from build123d import *

# Parameters (mm, degrees)
SKETCH1_R           = 7.875
BOSS_EXTRUDE1_DEPTH = 20.68
SKETCH2_R           = 8.915
BOSS_EXTRUDE2_DEPTH = 2.03
SKETCH3_R           = 5.965
SKETCH3_R_2         = 5.215
CUT_EXTRUDE1_DEPTH  = 0.4
CHAMFER1_SIZE       = 1.2
CHAMFER1_SIZE2      = 2.6
SKETCH4_R           = 5.34
BOSS_EXTRUDE3_DEPTH = 8.7
SKETCH5_W           = 0.4
SKETCH5_H           = 1.86
BOSS_EXTRUDE4_DEPTH = 5.65
SKETCH6_R           = 0.5
CUT_EXTRUDE2_DEPTH  = 14.552865697
FILLET1_R           = 2


with BuildPart() as part:
    # Sketch1 → Boss-Extrude1 (new body)
    with BuildSketch(Plane(origin=(0, 0, 0), x_dir=(0, 0, -1), z_dir=(1, 0, 0))):
        Circle(SKETCH1_R)
    extrude(amount=BOSS_EXTRUDE1_DEPTH)

    # Sketch2 → Boss-Extrude2 (add)
    with BuildSketch(Plane(origin=(20.68, 0, 0), x_dir=(0, 0, -1), z_dir=(1, 0, 0))):
        Circle(SKETCH2_R)
    extrude(amount=BOSS_EXTRUDE2_DEPTH)

    # Sketch3 → Cut-Extrude1 (cut)
    with BuildSketch(Plane(origin=(22.71, 0, 0), x_dir=(0, 0, -1), z_dir=(1, 0, 0))):
        Circle(SKETCH3_R)
        Circle(SKETCH3_R_2, mode=Mode.SUBTRACT)
    extrude(amount=-CUT_EXTRUDE1_DEPTH, mode=Mode.SUBTRACT)

    # Chamfer1
    chamfer1_edges = [part.edges().sort_by_distance(p)[0] for p in [
        (22.71, 0, 8.915),
    ]]
    chamfer1_side = [part.faces().sort_by_distance(p)[0] for p in [
        (21.695, 0, 8.915),
    ]]
    chamfer(chamfer1_edges, length=CHAMFER1_SIZE, length2=CHAMFER1_SIZE2, reference=chamfer1_side[0])

    # Sketch4 → Boss-Extrude3 (add)
    with BuildSketch(Plane.ZY):
        Circle(SKETCH4_R)
    extrude(amount=BOSS_EXTRUDE3_DEPTH)

    # Sketch5 → Boss-Extrude4 (add)
    with BuildSketch(Plane.ZY.offset(8.7)):
        with Locations((-2.90816811, 2.08596309)):
            Rectangle(SKETCH5_W, SKETCH5_H)
        with Locations((0, 2.08596309)):
            Rectangle(SKETCH5_W, SKETCH5_H)
        with Locations((2.90816811, 2.08596309)):
            Rectangle(SKETCH5_W, SKETCH5_H)
        with Locations((4.437865697, 0)):
            Rectangle(SKETCH5_W, SKETCH5_H)
        with Locations((-4.437865697, 0)):
            Rectangle(SKETCH5_W, SKETCH5_H)
    extrude(amount=BOSS_EXTRUDE4_DEPTH)

    # Sketch6 → Cut-Extrude2 (cut, through all)
    with BuildSketch(Plane(origin=(0, 0, -4.637865697), x_dir=(-1, 0, 0), z_dir=(0, 0, -1))):
        with Locations((13.385032673, 0)):
            Circle(SKETCH6_R)
        with Locations((13.385032673, 2.08596309)):
            Circle(SKETCH6_R)
    extrude(amount=-CUT_EXTRUDE2_DEPTH, mode=Mode.SUBTRACT)

    # Fillet1
    fillet1_edges = [part.edges().sort_by_distance(p)[0] for p in [
        (0, 0, 7.875),
    ]]
    fillet(fillet1_edges, radius=FILLET1_R)


solid = part.part
Verification items for the finished model (mm, model axes). A direction names the side the tool comes from. Give positions to 0.01 mm unless a question says otherwise; leave off trailing zeros. Loops run counter-clockwise (first coordinate to the right, second up) from the corner with the lowest first, then second, coordinate; pieces in that order, holes last.
1. Go/stop test with flat-tipped pins: P1, Ø4, axis at x = 3.5, z = -0.5, coming from the -Y side (3 decimals); P2, Ø5, axis at x = 13, z = -6, coming from the +Y side; P3, Ø1, axis at y = 5, z = -4.5, coming from the -X side. Record where each tip stops, or that it passes through.
Derived:
P1: stops at y = -7.875
P2: stops at y = 7.05
P3: stops at x = 0.03
2. Tool access check on faces 4 (the flat face through (20.68, -8, -1)), 5 (the cylindrical face through (22.513, -5.823, 1.293)), 6 (the flat face through (-11, 2, -3.108)), 7 (the flat face through (-11, 0, 4.238)), 8 (the flat face through (-11, 0, 4.638)). Record the directions out of +Z, -Z, +X, -X, +Y, -Y that give a thin tool (end or side, any length) a straight path to the whole face; none if there is none.
Derived:
face 4: -X
face 5: +X
face 6: -Z, -X, +Y, -Y
face 7: -X, +Y, -Y
face 8: +Z, -X, +Y, -Y
3. Release check for a two-part mould opening along Y. For faces 1 (the flat face through (22.31, -4, -4)), 2 (the cylindrical face through (-4.289, 0.235, -5.335)), 3 (the flat face through (-11, 0, -4.238)) record: +Y half, -Y half, draft (parallel to the pull), parting line (faces both ways), or undercut.
Derived:
face 1: undercut
face 2: parting line
face 3: draft
4. Cross-section at A-A on y = 0. Count the separate pieces of the cut face and the enclosed holes in it, and give its area (3 significant figures).
Derived:
separate pieces: 3
enclosed holes: 0
area: 453 mm2
5. Cross-section at C-C on x = -3. Record the cut outline in (y, z), and give its area (3 significant figures).
Derived:
outline: circle Ø10.68 at (0, 0)
area: 89.6 mm2
6. Cross-section at B-B on x = 9. Record the cut outline in (y, z) (3 decimals).
Derived:
outline: circle Ø15.75 at (0, 0)
7. Material ranges on probe 1 along X at (y, z) = (-2.25, -0.75); probe 2 along Y at (x, z) = (14, 0) (3 decimals); probe 3 along Y at (x, z) = (22.6, 0) (3 decimals), recorded low to high.
Derived:
probe 1: x = -8.7 to 22.71
probe 2: y = -7.875 to 7.875
probe 3: y = -6.553 to -5.965, -5.215 to 5.215, 5.965 to 6.553
